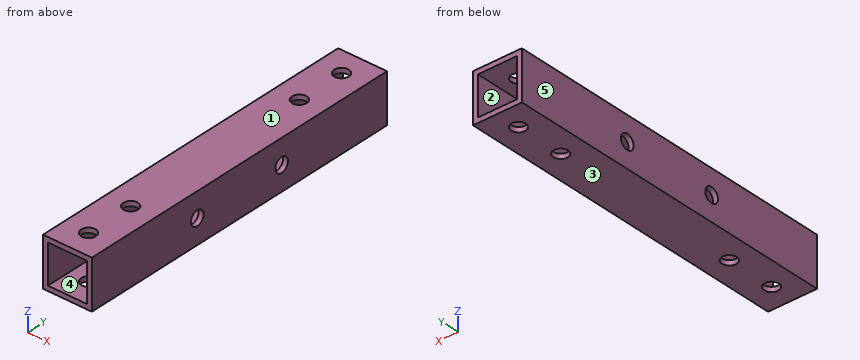
```python
from build123d import *

# Parameters (mm, degrees)
SKETCH_1_W          = 10
SKETCH_1_H          = 10
SKETCH_1_W_2        = 8
SKETCH_1_H_2        = 8
EXTRUDE_1_DEPTH     = 70
SKETCH_2_R          = 1.5
CUT_EXTRUDE_1_DEPTH = 30
SKETCH_3_R          = 1.5
CUT_EXTRUDE_2_DEPTH = 30


with BuildPart() as part:
    # 草图1 → 凸台-拉伸1 (new body)
    with BuildSketch(Plane(origin=(0, 0, 0), x_dir=(1, 0, 0), z_dir=(0, 1, 0))):
        Rectangle(SKETCH_1_W, SKETCH_1_H)
        Rectangle(SKETCH_1_W_2, SKETCH_1_H_2, mode=Mode.SUBTRACT)
    extrude(amount=EXTRUDE_1_DEPTH)

    # 草图2 → 切除-拉伸1 (cut)
    with BuildSketch(Plane.ZY.offset(5)):
        with Locations((0, 25)):
            Circle(SKETCH_2_R)
        with Locations((0, 45)):
            Circle(SKETCH_2_R)
    extrude(amount=-CUT_EXTRUDE_1_DEPTH, mode=Mode.SUBTRACT)

    # 草图3 → 切除-拉伸2 (cut)
    with BuildSketch(Plane(origin=(0, 0, -5), x_dir=(-1, 0, 0), z_dir=(0, 0, -1))):
        with Locations((0, 65)):
            Circle(SKETCH_3_R)
        with Locations((0, 55)):
            Circle(SKETCH_3_R)
        with Locations((0, 15)):
            Circle(SKETCH_3_R)
        with Locations((0, 5)):
            Circle(SKETCH_3_R)
    extrude(amount=-CUT_EXTRUDE_2_DEPTH, mode=Mode.SUBTRACT)


solid = part.part
```
The listing builds one solid part. Answer for the finished solid, in the listing's coordinates (mm). Face numbers are marked on the shaded views. A direction names the side the tool comes from. Give positions to 0.01 mm unless a question says otherwise; leave off trailing zeros. Order: outer loops, then holes, each group sorted by start corner. A loop starts at its lowest first (then second) coordinate and runs counter-clockwise, first axis right, second up. Notation, with made-up numbers: (6.25, 89) -> (62.25, 89) arc R13 cw to (62.25, 100) -> close; hole circle Ø7 at (-18.5, 22.25). An arc over 180 degrees is marked (long way). Write each question's results on one line, items separated by ' | '.
Q1. The part is cut by section C-C, the plane y = 30. Give the vertices of the cut face in (x, z).
Checked values:
outline: (-5, -5) -> (5, -5) -> (5, 5) -> (-5, 5) -> close; hole (-4, -4) -> (4, -4) -> (4, 4) -> (-4, 4) -> close
Q2. Straight lines are drawn through the part: probe 1 along Y at (x, z) = (4.2, 0); probe 2 along Y at (x, z) = (0, 4.7); probe 3 along Z at (x, y) = (2.25, 32). For each, find the intervals that lie inside material, in ascending order. Write a range as from..to.
Checked values:
probe 1: y = 0..23.5, 26.5..43.5, 46.5..70 | probe 2: y = 0..3.5, 6.5..13.5, 16.5..53.5, 56.5..63.5, 66.5..70 | probe 3: z = -5..-4, 4..5
Q3. The part is cut by section A-A, the plane y = 15. Give the vertices of the cut face in (x, z), and give its area (3 significant figures).
Checked values:
outline: (-5, -5) -> (-1.5, -5) -> (-1.5, -4) -> (-4, -4) -> (-4, 4) -> (-1.5, 4) -> (-1.5, 5) -> (-5, 5) -> close; (1.5, -5) -> (5, -5) -> (5, 5) -> (1.5, 5) -> (1.5, 4) -> (4, 4) -> (4, -4) -> (1.5, -4) -> close | area: 30.0 mm^2
Q4. The part is cut by section B-B, the plane z = 0. Give the vertices of the cut face in (x, y), and give its area (3 significant figures).
Checked values:
outline: (-5, 0) -> (-4, 0) -> (-4, 23.5) -> (-5, 23.5) -> close; (-5, 26.5) -> (-4, 26.5) -> (-4, 43.5) -> (-5, 43.5) -> close; (-5, 46.5) -> (-4, 46.5) -> (-4, 70) -> (-5, 70) -> close; (4, 0) -> (5, 0) -> (5, 23.5) -> (4, 23.5) -> close; (4, 26.5) -> (5, 26.5) -> (5, 43.5) -> (4, 43.5) -> close; (4, 46.5) -> (5, 46.5) -> (5, 70) -> (4, 70) -> close | area: 128 mm^2
Q5. The part is cut by section D-D, the plane x = -3. Give the vertices of the cut face in (y, z), and give its area (3 significant figures).
Checked values:
outline: (0, -5) -> (70, -5) -> (70, -4) -> (0, -4) -> close; (0, 4) -> (70, 4) -> (70, 5) -> (0, 5) -> close | area: 140 mm^2
Q6. Determine the mould class of the marked faces 3, 4 and 5 for opening direction X: pulls with the +X half, pulls with the -X half, needs draft (parallel to the pull), parting line crosses it, or undercut.
Checked values:
face 3: needs draft | face 4: undercut | face 5: pulls with the -X half
Q7. Which of the six approach directions +Z, -Z, +X, -X, +Y, -Y give full straight-line access (tool end or side, diameter ignored) to the marked faces 1 and 2?
Checked values:
face 1: +Z, +X, -X, +Y, -Y | face 2: +Y, -Y
